from build123d import *

# Parameters (mm, degrees)
SKETCH1_R           = 30
BOSS_EXTRUDE1_DEPTH = 40
SKETCH2_R           = 15
CUT_EXTRUDE1_DEPTH  = 11.5
SKETCH3_W           = 20
SKETCH3_H           = 30
BOSS_EXTRUDE2_DEPTH = 43.77
FILLET1_R           = 10
SKETCH4_R           = 7.5
CUT_EXTRUDE2_DEPTH  = 43.77
CUT_EXTRUDE3_DEPTH  = 1.85
CIRPATTERN1_COUNT   = 11


with BuildPart() as part:
    # Sketch1 → Boss-Extrude1 (new body)
    with BuildSketch(Plane.XY):
        Circle(SKETCH1_R)
    extrude(amount=-BOSS_EXTRUDE1_DEPTH)

    # Sketch2 → Cut-Extrude1 (cut)
    with BuildSketch(Plane.XY):
        Circle(SKETCH2_R)
    extrude(amount=-CUT_EXTRUDE1_DEPTH, mode=Mode.SUBTRACT)

    # Sketch3 → Boss-Extrude2 (add)
    with BuildSketch(Plane(origin=(0, 0, -40), x_dir=(-1, 0, 0), z_dir=(0, 0, -1))):
        Rectangle(SKETCH3_W, SKETCH3_H)
    extrude(amount=BOSS_EXTRUDE2_DEPTH)

    # Fillet1
    fillet1_edges = [part.edges().sort_by_distance(p)[0] for p in [
        (0, -15, -83.77),
        (0, 15, -83.77),
    ]]
    fillet(fillet1_edges, radius=FILLET1_R)

    # Sketch4 → Cut-Extrude2 (cut)
    with BuildSketch(Plane.ZY.offset(10)):
        with Locations(Location((-71.36, 0, 0), (0, 0, 270))):
            Circle(SKETCH4_R)
    extrude(amount=-CUT_EXTRUDE2_DEPTH, mode=Mode.SUBTRACT)

    # Sketch5 → Cut-Extrude3 (cut)
    with BuildSketch(Plane(origin=(0, 30, 0), x_dir=(1, 0, 0), z_dir=(0, 1, 0))):
        with BuildLine():
            Line((3, 35), (3, 5))
            ThreePointArc((3, 5), (0, 2), (-3, 5))
            Line((-3, 5), (-3, 35))
            ThreePointArc((-3, 35), (0, 38), (3, 35))
        make_face()
    cut_extrude3 = extrude(amount=-CUT_EXTRUDE3_DEPTH, mode=Mode.SUBTRACT)

    # CirPattern1: Cut-Extrude3 ×11 about axis
    cirpattern1_axis = Axis((0, 0, 0), (0, 0, 1))
    for i in range(1, CIRPATTERN1_COUNT):
        add(cut_extrude3.rotate(cirpattern1_axis, i * 360 / CIRPATTERN1_COUNT), mode=Mode.SUBTRACT)


solid = part.part
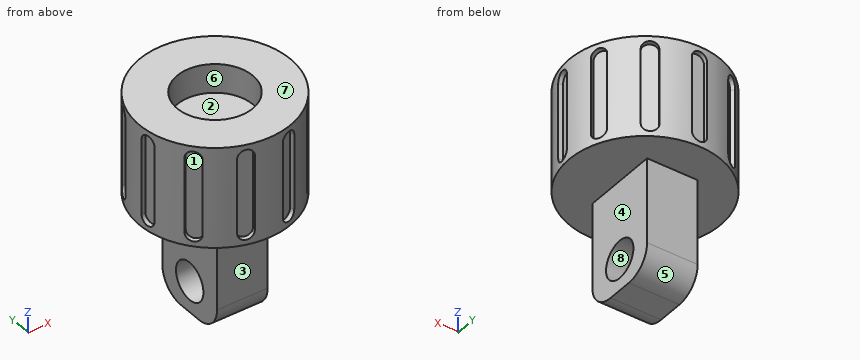
Model file for the job. Use its own axes, mm. Face numbers are marked on the shaded views. A direction names the side the tool comes from. Give positions to 0.01 mm unless a question says otherwise; leave off trailing zeros. Order: outer loops, then holes, each group sorted by start corner. A loop starts at its lowest first (then second) coordinate and runs counter-clockwise, first axis right, second up. Notation, with made-up numbers: (79.5, -33.75) - (130.5, -33.75) arc R22 cw to (130.5, 4.25) - close; hole circle Ø5 at (-8, 40). An arc over 180 degrees is marked (long way). Write item = value, one per line. Start each with the question number.
1. Probe line 1 along Z through (x, y) = (0.25, 0); line 2 along X through (y, z) = (2.5, -46.5); line 3 along Z through (x, y) = (-7.5, 15.5). List the from-to ranges inside material, lowest first.
2. Cut at D-D, the plane z = -44.5. List the corners of the cut face in (x, y), and give its area (3 significant figures).
3. Cut at B-B, the plane z = -71.36. List the corners of the cut face in (x, y), and give its area (3 significant figures).
4. Cut at C-C, the plane y = 1. List the corners of the cut face in (x, z), and give its area (3 significant figures).
5. Cut at A-A, the plane x = 0. List the corners of the cut face in (y, z), and give its area (3 significant figures).
6. Drop flat-ended pins along their axis: P1, Ø8, axis at y = -12, z = -51.5, coming from the -X side; P2, Ø10, axis at x = 1.5, z = -60.5, coming from the -Y side; P3, Ø1.5, axis at x = -13, y = 2.5, coming from the -Z side; P4, Ø1.5, axis at x = -4.5, y = 16, coming from the +Z side. Give the stop position or say it passes through.
7. Which spindle directions (+Z, -Z, +X, -X, +Y, -Y) get a long thin tool onto all of the face, cutting with end or side? Do the marked faces 1, 2, 3 and 4. Say none if no direction does.
8. Two-plate mould, pull along Y, no slides. Class the marked faces 5, 6, 7 and 8: pulls with the +Y half, pulls with the -Y half, needs draft (parallel to the pull), parting line crosses it, or undercut.
Taken from the geometry:
q1.line_1 = -83.77 to -78.86, -63.86 to -11.5
q1.line_2 = -10 to 10
q1.line_3 = -40 to 0
q2.outline = (-10, -15) - (10, -15) - (10, 15) - (-10, 15) - close
q2.area = 600 mm²
q3.outline = (-10, -15) - (10, -15) - (10, -7.5) - (-10, -7.5) - close; (-10, 7.5) - (10, 7.5) - (10, 15) - (-10, 15) - close
q3.area = 300 mm²
q4.outline = (-29.98, -40) - (-10, -40) - (-10, -63.93) - (10, -63.93) - (10, -40) - (29.98, -40) - (29.98, 0) - (14.97, 0) - (14.97, -11.5) - (-14.97, -11.5) - (-14.97, 0) - (-29.98, 0) - close; (-10, -83.77) - (10, -83.77) - (10, -78.79) - (-10, -78.79) - close
q4.area = 2,630 mm²
q5.outline = (-30, -40) - (-15, -40) - (-15, -73.77) arc R10 ccw to (-5, -83.77) - (5, -83.77) arc R10 ccw to (15, -73.77) - (15, -40) - (30, -40) - (30, -38) - (28.15, -38) - (28.15, -2) - (30, -2) - (30, 0) - (15, 0) - (15, -11.5) - (-15, -11.5) - (-15, 0) - (-30, 0) - close; hole circle Ø15 at (0, -71.36)
q5.area = 3,080 mm²
q6.P1 = -10
q6.P2 = -15
q6.P3 = -40
q6.P4 = 0
q7.face_1 = none
q7.face_2 = +Z
q7.face_3 = -Z, +X, -X, -Y
q7.face_4 = -Z, +X, +Y, -Y
q8.face_5 = pulls with the +Y half
q8.face_6 = undercut
q8.face_7 = needs draft
q8.face_8 = undercut
